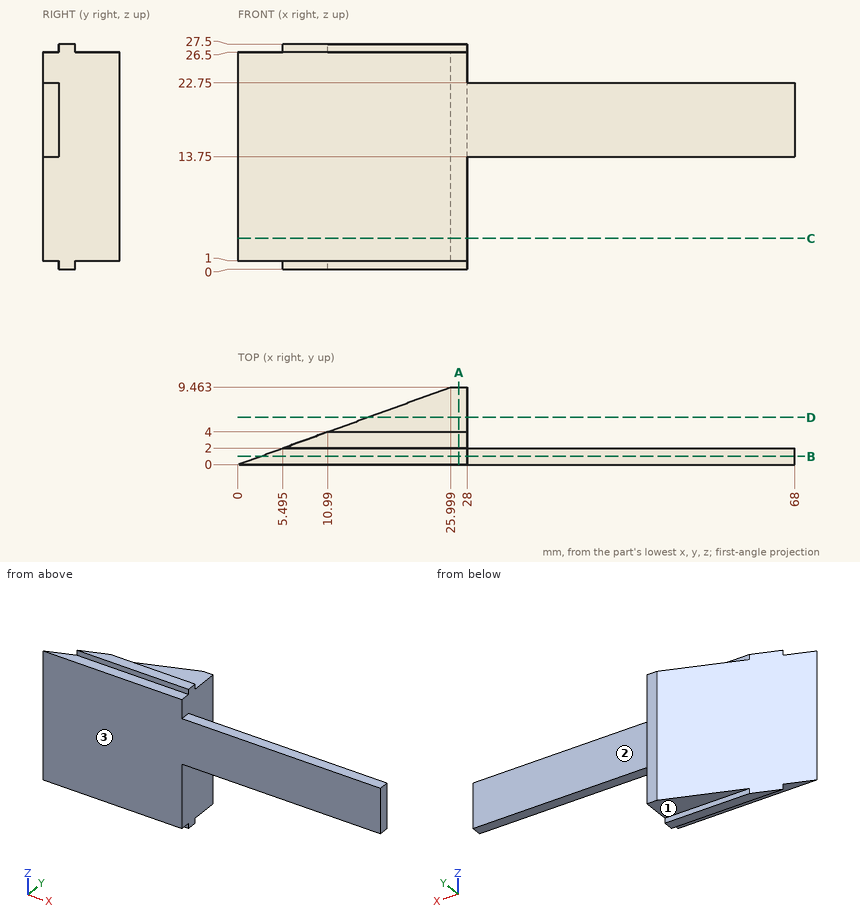
Could you check a few things on this drawing? It's one solid part, dimensions in mm from its lowest x, y, z. A direction names the side the tool comes from. Round coordinates to 2 decimals unless told otherwise and drop trailing zeros. Order: outer loops, then holes, each group sorted by start corner. A loop starts at its lowest first (then second) coordinate and runs counter-clockwise, first axis right, second up. Notation, with made-up numbers: M 69,-5.5 L 82,-5.5 A11 ccw 82,15.5 Z; hole C -28.75,-14 d9. An arc over 180 degrees is marked long. Use a Markdown table: item, result.
1) Imagine slicing it at A-A (x = 27). List the corners of the cut face in (y, z) for me, then the cut area to 3 significant figures.
Geometry says:
| item | result |
|---|---|
| outline | M 0,1 L 2,1 L 2,0 L 4,0 L 4,1 L 9.46,1 L 9.46,26.5 L 4,26.5 L 4,27.5 L 2,27.5 L 2,26.5 L 0,26.5 Z |
| area | 245 mm² |
2) Imagine slicing it at B-B (y = 1). List the corners of the cut face in (x, z) for me.
Geometry says:
| item | result |
|---|---|
| outline | M 2.75,1 L 28,1 L 28,13.75 L 68,13.75 L 68,22.75 L 28,22.75 L 28,26.5 L 2.75,26.5 Z |
3) I'm going to push flat-ended pins straight in: P1, Ø1.6, axis at x = 18.5, y = 0.5, coming from the +Z side; P2, Ø2.5, axis at x = 52.5, z = 18.5, coming from the +Y side; P3, Ø0.5, axis at x = 16, z = 27, coming from the +Y side. Where does each tip first touch, or does it pass through?
Geometry says:
| item | result |
|---|---|
| P1 | stops at z = 26.5 |
| P2 | stops at y = 2 |
| P3 | stops at y = 4 |
4) Imagine slicing it at D-D (y = 5.75). List the corners of the cut face in (x, z) for me, then the cut area to 3 significant figures.
Geometry says:
| item | result |
|---|---|
| outline | M 15.8,1 L 28,1 L 28,26.5 L 15.8,26.5 Z |
| area | 311 mm² |
5) If I drill on line 1 along Z through (x, y) = (27.5, 8.75); line 2 along Y through (x, z) = (36.5, 14); line 3 along Z through (x, y) = (64, 1.75), over which ranges is the centre line in solid material (lowest first)?
Geometry says:
| item | result |
|---|---|
| line 1 | z = 1 to 26.5 |
| line 2 | y = 0 to 2 |
| line 3 | z = 13.75 to 22.75 |
6) Imagine slicing it at C-C (z = 3.75). List the corners of the cut face in (x, y) for me.
Geometry says:
| item | result |
|---|---|
| outline | M 0,0 L 28,0 L 28,9.46 L 26,9.46 Z |
7) On a 3-axis mill with a long thin cutter (end or side, diameter ignored), from which of +Z, -Z, +X, -X, +Y, -Y can I reach the whole of each face in a straight line? I mean the marked faces 1, 2 and 3. Say none if no direction works.
Geometry says:
| item | result |
|---|---|
| face 1 | -Z, +X, -X, +Y |
| face 2 | +Z, -Z, +X, +Y |
| face 3 | +Z, -Z, +X, -X, -Y |
